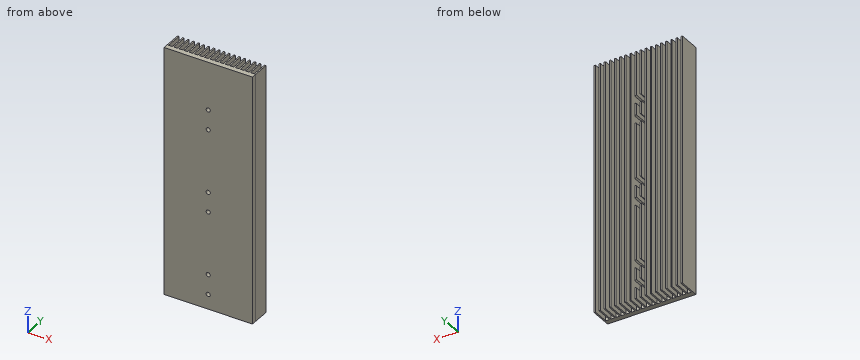
from build123d import *

# Parameters (mm, degrees)
SKETCH1_W          = 136.525
SKETCH1_H          = 381
EXTRUDE1_DEPTH     = 7.9248
SKETCH4_W          = 2.1844
SKETCH4_H          = 381
EXTRUDE2_DEPTH     = 25.4
LPATTERN1_COUNT    = 18
LPATTERN1_PITCH    = 7.902448
SKETCH6_R          = 3.175
CUT_EXTRUDE2_DEPTH = 10.16
SKETCH7_R          = 7.14375
CUT_EXTRUDE3_DEPTH = 406.518819594


with BuildPart() as part:
    # Sketch1 → Extrude1 (new body)
    with BuildSketch(Plane(origin=(0, 0, 0), x_dir=(1, 0, 0), z_dir=(0, 1, 0))):
        with Locations((68.2625, 190.5)):
            Rectangle(SKETCH1_W, SKETCH1_H)
    extrude(amount=EXTRUDE1_DEPTH)

    # Sketch4 → Extrude2 (add)
    with BuildSketch(Plane(origin=(0, 7.9248, 0), x_dir=(-1, 0, 0), z_dir=(0, 1, 0))):
        with Locations((-1.0922, -190.5)):
            Rectangle(SKETCH4_W, SKETCH4_H)
    extrude2 = extrude(amount=EXTRUDE2_DEPTH)

    # LPattern1: Extrude2 ×18
    with Locations(*[(i * LPATTERN1_PITCH, 0, 0) for i in range(1, LPATTERN1_COUNT)]):
        add(extrude2)

    # Sketch6 → Cut-Extrude2 (cut)
    with BuildSketch(Plane(origin=(0, 0, 0), x_dir=(1, 0, 0), z_dir=(0, 1, 0))):
        with Locations(Location((68.2625, 358.14, 0), (0, 0, 154.200161739))):
            Circle(SKETCH6_R)
        with Locations(Location((68.2625, 327.66, 0), (0, 0, 154.200161739))):
            Circle(SKETCH6_R)
        with Locations(Location((68.2625, 200.66, 0), (0, 0, 154.200161739))):
            Circle(SKETCH6_R)
        with Locations(Location((68.2625, 231.14, 0), (0, 0, 154.200161739))):
            Circle(SKETCH6_R)
        with Locations(Location((68.2625, 73.66, 0), (0, 0, 154.200161739))):
            Circle(SKETCH6_R)
        with Locations(Location((68.2625, 104.14, 0), (0, 0, 154.200161739))):
            Circle(SKETCH6_R)
    extrude(amount=CUT_EXTRUDE2_DEPTH, mode=Mode.SUBTRACT)

    # Sketch7 → Cut-Extrude3 (cut, through all)
    with BuildSketch(Plane(origin=(0, 7.9248, 0), x_dir=(-1, 0, 0), z_dir=(0, 1, 0))):
        with Locations((-68.2625, -358.14)):
            Circle(SKETCH7_R)
        with Locations((-68.2625, -327.66)):
            Circle(SKETCH7_R)
        with Locations((-68.2625, -231.14)):
            Circle(SKETCH7_R)
        with Locations((-68.2625, -200.66)):
            Circle(SKETCH7_R)
        with Locations((-68.2625, -73.66)):
            Circle(SKETCH7_R)
        with Locations((-68.2625, -104.14)):
            Circle(SKETCH7_R)
    extrude(amount=CUT_EXTRUDE3_DEPTH, mode=Mode.SUBTRACT)


solid = part.part
Could you check a few things on this model? Use its own coordinates, in mm. Give positions to 0.01 mm unless a question says otherwise; leave off trailing zeros.
1. For pin 1 (8.5 mm diameter, centred on y = 22.5, z = -91, fed in from -X); pin 2 (1.7 mm diameter, centred on x = 114.5, z = -222.5, fed in from +Y); pin 3 (1.5 mm diameter, centred on x = 36.5, y = 26.5, fed in from -Z), each with a flat end and sliding along its axis, tell me the tip position at first contact or that it passes through.
Answers below:
pin 1: stops at x = 0
pin 2: stops at y = 7.92
pin 3: passes through
2. I need wall thicknesses on L1, parallel to X at y = 2, z = -104 (3 decimals); L2, parallel to Y at x = 45.5, z = -330.5. Which ranges of each line are inside material? Lowest first, please.
Answers below:
L1: x = 0 to 65.091, 71.434 to 136.525
L2: y = 0 to 7.92
3. Suppose I cut it at A-A (y = 27.5). State how many separate pieces and enclosed holes the cut face has, plus the area to 3 significant figures.
Answers below:
separate pieces: 30
enclosed holes: 0
area: 14,700 mm2
